Autodesk Inventor part; units mm, degrees
ref_plane "YZ Plane" through (0, 0, 0) normal (1, 0, 0) x (0, 1, 0)
ref_plane "XZ Plane" through (0, 0, 0) normal (0, 1, 0) x (-1, 0, 0)
ref_plane "XY Plane" through (0, 0, 0) normal (0, 0, 1) x (1, 0, 0)
sketch "Sketch1" plane through (0, 0, 0) normal (0, 0, 1) x (1, 0, 0)
  circle A0 centre (0, 0) radius 3.25
  dimension "d0" = 6.5
extrude "Extrusion1" add sketch "Sketch1" along normal blind 70
sketch "Sketch2" plane through (0, 0, 70) normal (0, 0, 1) x (1, 0, 0)
  circle A0 centre (0, 0) radius 3.25
  circle A1 centre (0, 0) radius 2.5
  dimension "d3" = 5
extrude "Extrusion2" add sketch "Sketch2" along normal blind 10 contours A1
sketch "Sketch3" plane through (0, 0, 0) normal (0, 0, -1) x (-1, 0, 0)
  circle A0 centre (0, 0) radius 3.25
  circle A1 centre (0, 0) radius 2.5
  dimension "d6" = 5
extrude "Extrusion3" add sketch "Sketch3" along normal blind 7 contours A1
thread "Thread1"
thread "Thread2"
properties part number "18 - Piston Rod" material "Steel AISI 1020 107 HR"
Can you work these out from the model? Positions are in its coordinate system, mm. A direction names the side the tool comes from. Coordinates: 2 decimals unless noted, no trailing zeros. Write each loop counter-clockwise with the first axis right and the second up, starting at its lowest first coordinate (ties: lowest second). Pieces come first, ordered by that corner, then holes. Notation, with made-up numbers: M 34,-37.5 L 43,-37.5 A27 ccw 43,-21.5 Z; hole C 37.25,32 d3. An arc over 180 degrees is marked long. Use one line per item in the form item = value.
Q1. If we section it at C-C (z = 65): Write out the boundary of the cut face in (x, y), then the cut area to 3 significant figures.
Model answer:
outline = C 0,0 d6.5
area = 33.2 mm^2
Q2. I need wall thicknesses on line 1 along Z through (x, y) = (0.25, 3); line 2 along Y through (x, z) = (1.75, 17); line 3 along Y through (x, z) = (-0.5, 19). Which ranges of each line are inside material? Lowest first, please. Write a range as from..to.
Model answer:
line_1 = 0..70
line_2 = -2.74..2.74
line_3 = -3.21..3.21
Q3. For faces 1 (the flat face through (2, -2, 70)), 2 (the cylindrical face through (-2.579, 1.978, 34.51)), 3 (the cylindrical face through (0.54, 2.44, -3.45)), which set-ups out of +Z, -Z, +X, -X, +Y, -Y let a thin tool reach every point of the face, with its end or its side?
Model answer:
face_1 = +Z
face_2 = +Z, -Z
face_3 = -Z
Q4. If we section it at A-A (y = 0): Write out the boundary of the cut face in (x, z), then the cut area to 3 significant figures.
Model answer:
outline = M -3.25,0 L -2.5,0 L -2.5,-7 L 2.5,-7 L 2.5,0 L 3.25,0 L 3.25,70 L 2.5,70 L 2.5,80 L -2.5,80 L -2.5,70 L -3.25,70 Z
area = 540 mm^2
Q5. For P1, Ø2, axis at x = 1.5, z = 56, coming from the +Y side; P2, Ø1.5, axis at y = -2.5, z = 16, coming from the +X side; P3, Ø1, axis at y = 2.5, z = 61.5, coming from the -X side, each with a flat end and sliding along its axis, tell me the tip position at first contact or that it passes through.
Model answer:
P1 = 3.21
P2 = 2.74
P3 = -2.56
